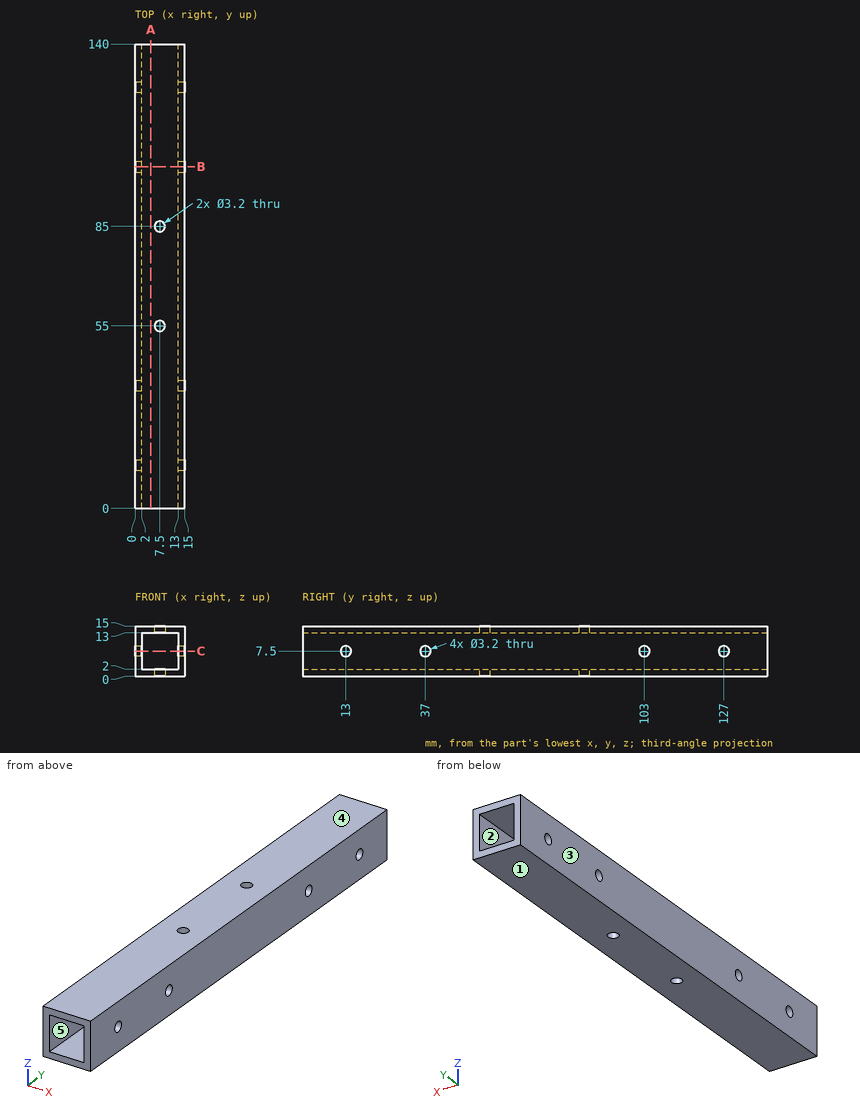
Drawing for the job (mm, zero at the part's lowest x, y, z). A direction names the side the tool comes from. Round coordinates to 2 decimals unless told otherwise and drop trailing zeros. Order: outer loops, then holes, each group sorted by start corner. A loop starts at its lowest first (then second) coordinate and runs counter-clockwise, first axis right, second up. Notation, with made-up numbers: (64.25, 70) -> (96.25, 70) arc R28 ccw to (96.25, 104) -> close; hole circle Ø5 at (50.25, 87). An arc over 180 degrees is marked (long way). Write item = value, one per line. Start each with the question number.
(1) Cut at C-C, the plane z = 7.5. State how many separate pieces and enclosed holes the cut face has, then the cut area to 3 significant figures.
(2) Probe line 1 (Y direction, x = 7.5, z = 0.7); line 2 (X direction, y = 67.5, z = 6.5). List the from-to ranges inside material, lowest first. Write a range as [from, to].
(3) Which spindle directions (+Z, -Z, +X, -X, +Y, -Y) get a long thin tool onto all of the face, cutting with end or side? Do the marked faces 4 and 5. Say none if no direction does.
(4) Cut at B-B, the plane y = 103. List the corners of the cut face in (x, z), then the cut area to 3 significant figures.
(5) Cut at A-A, the plane x = 4.75. List the corners of the cut face in (y, z), then the cut area to 3 significant figures.
(6) Pull direction X, two halves, no side cores. Call the marked faces 1, 2 and 3: released by +X, released by -X, zero draft, split by the parting line, or undercut.
Model answer:
q1.separate_pieces = 10
q1.enclosed_holes = 0
q1.area = 509 mm2
q2.line_1 = [0, 53.4], [56.6, 83.4], [86.6, 140]
q2.line_2 = [0, 2], [13, 15]
q3.face_4 = +Z, +X, -X, +Y, -Y
q3.face_5 = +Y, -Y
q4.outline = (0, 0) -> (15, 0) -> (15, 5.9) -> (13, 5.9) -> (13, 2) -> (2, 2) -> (2, 5.9) -> (0, 5.9) -> close; (0, 9.1) -> (2, 9.1) -> (2, 13) -> (13, 13) -> (13, 9.1) -> (15, 9.1) -> (15, 15) -> (0, 15) -> close
q4.area = 91.2 mm2
q5.outline = (0, 0) -> (140, 0) -> (140, 2) -> (0, 2) -> close; (0, 13) -> (140, 13) -> (140, 15) -> (0, 15) -> close
q5.area = 560 mm2
q6.face_1 = zero draft
q6.face_2 = undercut
q6.face_3 = released by -X
